Part model, mm, in its own coordinate system. A direction names the side the tool comes from. Give positions to 0.01 mm unless a question says otherwise; leave off trailing zeros. Write each loop counter-clockwise with the first axis right and the second up, starting at its lowest first coordinate (ties: lowest second). Pieces come first, ordered by that corner, then holes. Notation, with made-up numbers: M -0.5,-10.75 L 13.5,-10.75 A25 ccw 13.5,19.25 Z; hole C 51.25,-39 d7. An arc over 180 degrees is marked long. Use a Markdown table: item, result. Add a question column.
from build123d import *

# Parameters (mm, degrees)
FILLET1_R   = 2.54
SKETCH3_W   = 20.447112079
SKETCH3_H   = 3.175
SKETCH3_W_2 = 12.7


with BuildPart() as part:
    # Sketch2 → Revolve1 (revolve)
    with BuildSketch(Plane.XY, mode=Mode.PRIVATE) as revolve1_sk:
        Polygon((48.26, 0), (48.26, 76.2), (31.75, 76.2), (6.35, 40.64), (46.99, 0), align=None)
    revolve(revolve1_sk.sketch.rotate(Axis((0, 0, 0), (0, 1, 0)), 90), axis=Axis((0, 0, 0), (0, 1, 0)))

    # Fillet1
    fillet1_edges = [part.edges().sort_by_distance(p)[0] for p in [
        (0, 40.64, 6.35),
    ]]
    fillet(fillet1_edges, radius=FILLET1_R)

    # Sketch3 → Cut-Revolve1 (revolve, cut)
    with BuildSketch(Plane.XY, mode=Mode.PRIVATE) as cut_revolve1_sk:
        with Locations((55.30855604, 61.9125)):
            Rectangle(SKETCH3_W, SKETCH3_H)
        with Locations((51.435, 46.0375)):
            Rectangle(SKETCH3_W_2, SKETCH3_H)
    revolve(cut_revolve1_sk.sketch.rotate(Axis((0, 0, 0), (0, -1, 0)), 90), axis=Axis((0, 0, 0), (0, -1, 0)), mode=Mode.SUBTRACT)


solid = part.part
1. Tool access for faces 1 (the flat face through (46.2, 0, 10.5)), 2 (the flat face through (-22, 47.625, 40)): list every direction of +Z, -Z, +X, -X, +Y, -Y with a clear straight run to the whole face (end or side of a thin tool).
2. Mould opens along Z. For faces 3 (the cylindrical face through (-14.5, 69.94, -46.03)), 4 (the conical face through (-4.405, 32.325, -13.988)), 5 (the flat face through (-22, 60.325, 40)) say: released by +Z, released by -Z, zero draft, split by the parting line, or undercut.
3. Flat gauge pins, fed straight in: pin 1 (5 mm diameter, centred on x = 0, z = -23.5, fed in from +Y); pin 2 (12 mm diameter, centred on y = 52.5, z = 30.5, fed in from -X); pin 3 (2 mm diameter, centred on y = 10.5, z = 36.5, fed in from +X). Where does each tip first touch, or does it go through?
4. Drill centre lines: probe 1 along Y at (x, z) = (-28, -36) (3 decimals); probe 2 along Z at (x, y) = (-14.5, 69.5); probe 3 along X at (y, z) = (12.5, 17). Where is each one in solid material? Low to high. Write a range as [from, to].
5. Cut at B-B (y = 6.5). Write the cut outline in (x, z), then the cut area to 3 significant figures.
6. Cut at A-A (y = 27). Write the cut outline in (x, z).
A:
| question | item | result |
|---|---|---|
| 1 | face 1 | +Z, -Z, +X, -X, -Y |
| 1 | face 2 | none |
| 2 | face 3 | split by the parting line |
| 2 | face 4 | undercut |
| 2 | face 5 | zero draft |
| 3 | pin 1 | stops at y = 68.15 |
| 3 | pin 2 | stops at x = -41.58 |
| 3 | pin 3 | stops at x = 32.69 |
| 4 | probe 1 | y = [1.383, 44.45], [47.625, 60.325], [63.5, 76.2] |
| 4 | probe 2 | z = [-46.03, -22.73], [22.73, 46.03] |
| 4 | probe 3 | x = [-45.17, -30.01], [30.01, 45.17] |
| 5 | outline | C 0,0 d96.52; hole C 0,0 d80.98 |
| 5 | area | 2,170 mm² |
| 6 | outline | C 0,0 d96.52; hole C 0,0 d39.98 |
